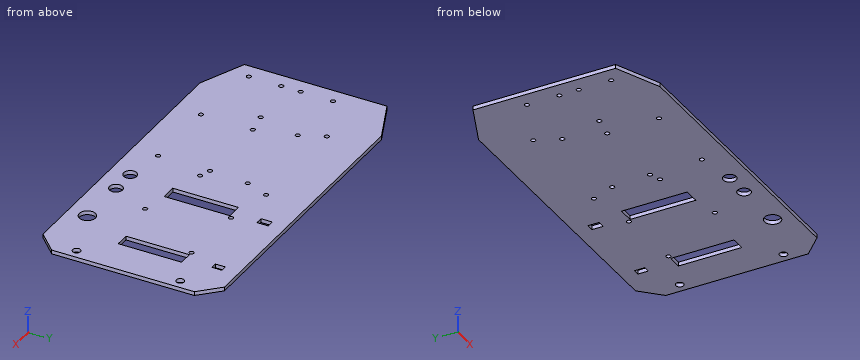
from build123d import *

# Parameters (mm, degrees)
SKETCH1_W           = 270
SKETCH1_H           = 140
BOSS_EXTRUDE1_DEPTH = 3
SKETCH2_R           = 6.25
SKETCH2_R_2         = 5
CUT_EXTRUDE1_DEPTH  = 3
CUT_EXTRUDE3_DEPTH  = 3
SKETCH6_W           = 12.019056062
SKETCH6_H           = 50.71745121
SKETCH6_W_2         = 10.934400461
SKETCH6_H_2         = 48.883202059
SKETCH6_W_3         = 5.676391459
SKETCH6_H_3         = 8.689402458
SKETCH6_W_4         = 4.853726277
SKETCH6_H_4         = 7.896916359
CUT_EXTRUDE5_DEPTH  = 10
SKETCH7_R           = 1.75
CUT_EXTRUDE8_DEPTH  = 10
SKETCH8_R           = 1.75
CUT_EXTRUDE9_DEPTH  = 10
SKETCH9_R           = 1.75
SKETCH9_R_2         = 3
CUT_EXTRUDE10_DEPTH = 10
SKETCH10_R          = 1.75
CUT_EXTRUDE11_DEPTH = 10


with BuildPart() as part:
    # Sketch1 → Boss-Extrude1 (new body)
    with BuildSketch(Plane.XY):
        with Locations((135, 70)):
            Rectangle(SKETCH1_W, SKETCH1_H)
    extrude(amount=BOSS_EXTRUDE1_DEPTH)

    # Sketch2 → Cut-Extrude1 (cut)
    with BuildSketch(Plane.XY.offset(3)):
        with Locations((220, 15)):
            Circle(SKETCH2_R)
        with Locations((180, 15)):
            Circle(SKETCH2_R_2)
        with Locations((160, 15)):
            Circle(SKETCH2_R_2)
    extrude(amount=-CUT_EXTRUDE1_DEPTH, mode=Mode.SUBTRACT)

    # Sketch5 → Cut-Extrude3 (cut)
    with BuildSketch(Plane.XY.offset(3)):
        Polygon((255, 140), (270, 125), (270, 140), align=None)
        Polygon((0, 140), (0, 125), (35, 140), align=None)
        Polygon((270, 0), (255, 0), (270, 15), align=None)
        Polygon((0, 15), (35, 0), (0, 0), align=None)
    extrude(amount=-CUT_EXTRUDE3_DEPTH, mode=Mode.SUBTRACT)

    # Sketch6 → Cut-Extrude5 (cut)
    with BuildSketch(Plane(origin=(0, 0, 0), x_dir=(-1, 0, 0), z_dir=(0, 0, -1))):
        with Locations((-167.493263023, 73.985112913)):
            Rectangle(SKETCH6_W, SKETCH6_H)
        with Locations((-235.732393676, 74.902237489)):
            Rectangle(SKETCH6_W_2, SKETCH6_H_2)
        with Locations((-169.594169913, 123.903401406)):
            Rectangle(SKETCH6_W_3, SKETCH6_H_3)
        with Locations((-234.619547555, 124.299644456)):
            Rectangle(SKETCH6_W_4, SKETCH6_H_4)
    extrude(amount=-CUT_EXTRUDE5_DEPTH, mode=Mode.SUBTRACT)

    # Sketch7 → Cut-Extrude8 (cut)
    with BuildSketch(Plane(origin=(0, 0, 0), x_dir=(-1, 0, 0), z_dir=(0, 0, -1))):
        with Locations((-53.483734992, 57)):
            Circle(SKETCH7_R)
        with Locations((-138.483734992, 57)):
            Circle(SKETCH7_R)
        with Locations((-138.483734992, 108)):
            Circle(SKETCH7_R)
        with Locations((-53.483734992, 108)):
            Circle(SKETCH7_R)
    extrude(amount=-CUT_EXTRUDE8_DEPTH, mode=Mode.SUBTRACT)

    # Sketch8 → Cut-Extrude9 (cut)
    with BuildSketch(Plane(origin=(0, 0, 0), x_dir=(-1, 0, 0), z_dir=(0, 0, -1))):
        with Locations((-12, 25)):
            Circle(SKETCH8_R)
        with Locations((-12, 65)):
            Circle(SKETCH8_R)
        with Locations((-12, 50)):
            Circle(SKETCH8_R)
        with Locations((-12, 90)):
            Circle(SKETCH8_R)
    extrude(amount=-CUT_EXTRUDE9_DEPTH, mode=Mode.SUBTRACT)

    # Sketch9 → Cut-Extrude10 (cut)
    with BuildSketch(Plane(origin=(0, 0, 0), x_dir=(-1, 0, 0), z_dir=(0, 0, -1))):
        with Locations((-70, 20)):
            Circle(SKETCH9_R)
        with Locations((-130, 20)):
            Circle(SKETCH9_R)
        with Locations((-130, 60)):
            Circle(SKETCH9_R)
        with Locations((-70, 60)):
            Circle(SKETCH9_R)
        with Locations((-61.483734992, 90)):
            Circle(SKETCH9_R)
        with Locations((-131.483734992, 90)):
            Circle(SKETCH9_R)
        with Locations((-262.5, 30)):
            Circle(SKETCH9_R_2)
        with Locations((-262.5, 110)):
            Circle(SKETCH9_R_2)
    extrude(amount=-CUT_EXTRUDE10_DEPTH, mode=Mode.SUBTRACT)

    # Sketch10 → Cut-Extrude11 (cut)
    with BuildSketch(Plane(origin=(0, 0, 0), x_dir=(-1, 0, 0), z_dir=(0, 0, -1))):
        with Locations((-193.502791054, 45)):
            Circle(SKETCH10_R)
        with Locations((-175.502791054, 101.343838518)):
            Circle(SKETCH10_R)
        with Locations((-227.265193445, 99.343838518)):
            Circle(SKETCH10_R)
    extrude(amount=-CUT_EXTRUDE11_DEPTH, mode=Mode.SUBTRACT)


solid = part.part
For this review, take the finished solid that the model builds, in its own axes (mm). Coordinates: 2 decimals unless noted, no trailing zeros. Write each loop counter-clockwise with the first axis right and the second up, starting at its lowest first coordinate (ties: lowest second). Pieces come first, ordered by that corner, then holes. Notation, with made-up numbers: (50.25, -16.75) -> (84.25, -16.75) arc R28 ccw to (84.25, 7.25) -> close; hole circle Ø8 at (13.25, 83.25). An arc over 180 degrees is marked (long way). Write each question's results on one line, items separated by ' | '. Start each with the question number.
1) Consider section B-B (z = 0.8). Give the number of separate pieces and of enclosed holes in the cut face, plus the area to 3 significant figures.
2) Wall thickness on L1, parallel to Y at x = 171.5, z = 0.6; L2, parallel to X at y = 99, z = 1.35; L3, parallel to Y at x = 71, z = 0.6: over which ranges is each line inside the solid? List them lowest first. Write a range as [from, to].
3) Consider section A-A (x = 262.5). Write out the cut boundary in (y, z), plus the area to 3 significant figures.
Geometry says:
1) separate pieces: 1 | enclosed holes: 26 | area: 35,300 mm^2
2) L1: [0, 48.63], [99.34, 119.56], [128.25, 140] | L2: [0, 161.48], [173.5, 225.55], [228.98, 230.27], [241.2, 270] | L3: [0, 18.56], [21.44, 58.56], [61.44, 140]
3) outline: (7.5, 0) -> (27, 0) -> (27, 3) -> (7.5, 3) -> close; (33, 0) -> (107, 0) -> (107, 3) -> (33, 3) -> close; (113, 0) -> (132.5, 0) -> (132.5, 3) -> (113, 3) -> close | area: 339 mm^2
